Source: CAD feature listing. Evaluate the final solid. Frame: model axes, mm. A direction names the side the tool comes from. Round coordinates to 2 decimals unless told otherwise and drop trailing zeros. Order: outer loops, then holes, each group sorted by start corner. A loop starts at its lowest first (then second) coordinate and runs counter-clockwise, first axis right, second up. Notation, with made-up numbers: (-10, -16) -> (-1, -16) arc R19 cw to (-1, 8) -> close; hole circle Ø3 at (59.25, 70.25). An arc over 180 degrees is marked (long way). Answer as CSV lines item,"result".
from build123d import *

# Parameters (mm, degrees)
EXTRUDE_1_DEPTH           = 20
HOLE_WIZARD_0_D           = 5.5
HOLE_WIZARD_0_CBORE_D     = 10
HOLE_WIZARD_0_CBORE_DEPTH = 5.7
HOLE_WIZARD_M4_1_D        = 3.3


with BuildPart() as part:
    # 草图1 → 凸台-拉伸1 (new body)
    with BuildSketch(Plane(origin=(0, 0, 0), x_dir=(1, 0, 0), z_dir=(0, 1, 0))):
        Polygon((-42.5, 24), (-29.5, 24), (-29.5, 8), (29.5, 8), (29.5, 24), (42.5, 24), (42.5, 0), (-42.5, 0), align=None)
    extrude(amount=EXTRUDE_1_DEPTH)

    # 打孔尺寸(%根据)内六角圆柱头螺钉的类型0 (through all)
    with Locations(Plane.XY):
        with Locations((19.5, 10), (-19.5, 10)):
            CounterBoreHole(HOLE_WIZARD_0_D / 2, HOLE_WIZARD_0_CBORE_D / 2, HOLE_WIZARD_0_CBORE_DEPTH)

    # M4 螺纹孔1 (through all)
    with Locations(Plane(origin=(0, 0, 0), x_dir=(-1, 0, 0), z_dir=(0, -1, 0))):
        with Locations((36, 4), (-36, 4), (36, 20), (-36, 20)):
            Hole(HOLE_WIZARD_M4_1_D / 2)


solid = part.part
1. Section query C-C on y = 18.5. Return loops of the section in (x, z), and give its area (3 significant figures).
Results below:
outline,"(-42.5, -24) -> (-29.5, -24) -> (-29.5, -8) -> (29.5, -8) -> (29.5, -24) -> (42.5, -24) -> (42.5, 0) -> (-42.5, 0) -> close; hole circle Ø3.3 at (-36, -20); hole circle Ø3.3 at (-36, -4); hole circle Ø3.3 at (36, -20); hole circle Ø3.3 at (36, -4)"
area,"1,060 mm2"
2. Section query D-D on z = -10.75. Return loops of the section in (x, y).
Results below:
outline,"(-42.5, 0) -> (-29.5, 0) -> (-29.5, 20) -> (-42.5, 20) -> close; (29.5, 0) -> (42.5, 0) -> (42.5, 20) -> (29.5, 20) -> close"
3. Line query: L1, parallel to Z at x = -36, y = 8.5; L2, parallel to X at y = 14.25, z = -20; L3, parallel to Y at x = 19.5, z = -1.9. Output: solid intervals per line, ascending. Write a range as [from, to].
Results below:
L1,"[-24, -21.65], [-18.35, -5.65], [-2.35, 0]"
L2,"[-42.5, -37.65], [-34.35, -29.5], [29.5, 34.35], [37.65, 42.5]"
L3,"[0, 5], [15, 20]"
4. Mould query, pull axis Z, two halves, no side actions, for faces 4 (the flat face through (36, 10, -24)), 5 (the flat face through (1, 20, -7)), 6 (the cylindrical face through (34.35, 10.14, -20.07)). Classes: released by +Z, released by -Z, zero draft, split by the parting line, or undercut.
Results below:
face 4,"released by -Z"
face 5,"zero draft"
face 6,"undercut"
5. Section query A-A on z = -4. Return loops of the section in (x, y).
Results below:
outline,"(-42.5, 0) -> (-37.65, 0) -> (-37.65, 20) -> (-42.5, 20) -> close; (-34.35, 0) -> (34.35, 0) -> (34.35, 20) -> (-34.35, 20) -> close; (37.65, 0) -> (42.5, 0) -> (42.5, 20) -> (37.65, 20) -> close; hole circle Ø10 at (-19.5, 10); hole circle Ø10 at (19.5, 10)"
6. Reachability of faces 1 (the flat face through (0, 10, -8)), 2 (the cylindrical face through (18.849, 14.957, -2.81)), 3 (the cylindrical face through (-17.473, 11.859, -6.866)) from +Z, -Z, +X, -X, +Y, -Y: full face, straight path, thin tool, end or side. Return the list, or none.
Results below:
face 1,"-Z, +Y, -Y"
face 2,"+Z"
face 3,"+Z, -Z"
7. Pin query (flat end, axial travel): pin 1 (6.5 mm diameter, centred on x = 19.5, y = 10, fed in from +Z); pin 2 (10 mm diameter, centred on x = 4.5, y = 12, fed in from -Z); pin 3 (2 mm diameter, centred on x = -30, y = 8.5, fed in from +Z). Return the tip coordinate at first contact, or that it passes through.
Results below:
pin 1,"z = -5.7"
pin 2,"z = -8"
pin 3,"z = 0"
8. Section query B-B on x = 19.5. Return loops of the section in (y, z), and give its area (4 significant figures).
Results below:
outline,"(0, -8) -> (7.25, -8) -> (7.25, -5.7) -> (5, -5.7) -> (5, 0) -> (0, 0) -> close; (12.75, -8) -> (20, -8) -> (20, 0) -> (15, 0) -> (15, -5.7) -> (12.75, -5.7) -> close"
area,"90.35 mm2"
